Source: CAD feature listing. Evaluate the final solid. Frame: model axes, mm. Coordinates: 2 decimals unless noted, no trailing zeros. Order: outer loops, then holes, each group sorted by start corner. A loop starts at its lowest first (then second) coordinate and runs counter-clockwise, first axis right, second up.
Item 1: Section A-A on x = 0. Return the cut outline in (y, z), then the cut area to 3 significant figures.
Item 2: Section D-D on y = 101. Return the cut outline in (x, z).
Item 3: Section B-B on z = 3.5. State how many separate pieces and enclosed holes the cut face has, then the cut area to 3 significant figures.
Item 4: Section C-C on y = 0. Return the cut outline in (x, z).
Item 5: Mould query, pull axis Y, two halves, no side actions, for faces 1 (the cylindrical face through (6.154, -1.938, 3.131)), 2 (the cylindrical face through (-49.938, 320.133, 3.131)), 3 (the flat face through (-44, 161, 6.35)), 4 (the flat face through (-92.426, 381.018, 3.131)). Classes: released by +Y, released by -Y, zero draft, split by the parting line, or undercut.
Item 6: Ray query, line 1 (Y direction, x = -30, z = 4.75); line 2 (X direction, y = 71.5, z = 0.75); line 3 (X direction, y = 330.5, z = 2). Return the intervals inside material, ascending.
Autodesk Inventor part; units mm, degrees
ref_plane "Work Plane1" through (-0.0003, 0.0023, 0) normal (0, 0, 1) x (1, 0, 0)
ref_plane "YZ Plane" through (0, 0, 0) normal (1, 0, 0) x (0, 1, 0)
ref_plane "XZ Plane" through (0, 0, 0) normal (0, 1, 0) x (-1, 0, 0)
ref_plane "Work Plane1" through (-0.0003, 0.0023, 0) normal (0, 0, 1) x (1, 0, 0)
sketch "Sketch1" plane through (-0.0003, 0.0023, 0) normal (0, 0, 1) x (1, 0, 0)
  circle A0 centre (0.0003, -0.0023) radius 6.3373 construction
  circle A1 centre (-49.0975, 326.5271) radius 6.3373 construction
  circle A2 centre (0.0003, -0.0023) radius 6.4516
  circle A3 centre (-49.0975, 326.5271) radius 6.4516
  circle A4 centre (-49.0975, 326.5271) radius 60.325 construction
  circle A5 centre (0.0003, -0.0023) radius 60.325 construction
  circle A6 centre (0.0003, -0.0023) radius 31.75 construction
  line L0 (40.3672, -54.9357) -> (-26.6702, 390.9025)
  circle A7 centre (-49.0975, 326.5271) radius 31.75 construction
  line L1 (-58.7973, -69.8464) -> (40.3672, -54.9357)
  line L2 (-125.8347, 375.9918) -> (-26.6702, 390.9025)
  circle A8 centre (-54.0299, 68.9302) radius 6.3373 construction
  circle A9 centre (-36.6118, 251.3479) radius 6.3373 construction
  circle A10 centre (-54.0299, 68.9302) radius 6.4516
  line L3 (-82.6344, 131.3852) -> (-87.6899, 165.0073) construction
  line L4 (-58.7973, -69.8464) -> (-125.8347, 375.9918)
  point P0 (0.0003, -0.0023)
  dimension "d0" = 12.9032
  dimension "d3" = 12.9032
  dimension "d11" = 120.65
  dimension "d13" = 120.65
  dimension "d14" = 63.5
  dimension "d16" = 63.5
  dimension "d19" = 12.9032
extrude "Extrusion1" add sketch "Sketch1" along normal blind 6.35
sketch "Sketch2" plane through (-0.0003, 0.0023, 0) normal (0, 0, -1) x (-1, 0, 0)
  circle A0 centre (111.3879, 365.3242) radius 1.778 construction
  circle A1 centre (77.9428, 262.471) radius 1.778 construction
  circle A2 centre (31.0502, 180.1901) radius 1.778 construction
  circle A3 centre (64.857, 175.1068) radius 1.778 construction
  circle A4 centre (25.7636, 145.0307) radius 1.778 construction
  circle A5 centre (59.5704, 139.9475) radius 1.778 construction
  circle A6 centre (48.1268, -55.3992) radius 1.778 construction
  circle A7 centre (111.3879, 365.3242) radius 1.778
  circle A8 centre (77.9428, 262.471) radius 1.778
  circle A9 centre (64.857, 175.1068) radius 1.778
  circle A10 centre (59.5704, 139.9475) radius 1.778
  circle A11 centre (31.0502, 180.1901) radius 1.778
  circle A12 centre (25.7636, 145.0307) radius 1.778
  circle A13 centre (48.1268, -55.3992) radius 1.778
  point P0 (-0.0003, -0.0023)
extrude "Extrusion2" cut sketch "Sketch2" against normal through all
sketch "Sketch3" plane through (-0.0003, 0.0023, 0) normal (0, 0, -1) x (-1, 0, 0)
  circle A0 centre (-7.8664, -5.812) radius 2.8702 construction
  circle A1 centre (58.7683, 60.3758) radius 2.8702 construction
  circle A2 centre (41.3502, 242.7936) radius 2.8702
  circle A3 centre (41.2314, 320.7173) radius 2.8702 construction
  circle A4 centre (39.1236, 318.7692) radius 2.9567
  circle A5 centre (42.9235, 240.393) radius 2.8702
  circle A6 centre (60.507, 58.0922) radius 2.8702
  circle A7 centre (-10.0879, -7.6295) radius 2.8702
  point P0 (-0.0003, -0.0023)
extrude "Extrusion3" cut sketch "Sketch3" against normal through all contours A2 A5 | A2 A5 | A4 | A6 | A7 picked at (41.9477, 242.03) picked at (43.9052, 238.7756)
sketch "Sketch4" plane through (-0.0003, 0.0023, 0) normal (0, 0, -1) x (-1, 0, 0)
  arc A0 (58.0673, 386.1815) -> (21.1234, 354.0125) centre (58.7307, 348.1214) ccw construction
  arc A1 (58.0673, 386.1815) -> (21.1234, 354.0125) centre (58.7307, 348.1214) ccw
  line L0 (26.6702, 390.9025) -> (125.8347, 375.9918)
  line L1 (58.0673, 386.1815) -> (26.6702, 390.9025)
  line L2 (26.6702, 390.9025) -> (21.1234, 354.0125)
  point P0 (-0.0003, -0.0023)
extrude "Extrusion4" cut sketch "Sketch4" against normal through all
sketch "Sketch5" plane through (-0.0003, 0.0023, 0) normal (0, 0, -1) x (-1, 0, 0)
  circle A0 centre (-9.1502, 60.0002) radius 2.25 construction
  circle A1 centre (-9.1502, 60.0002) radius 1.8542
  point P0 (-0.0003, -0.0023)
  dimension "d30" = 3.7084
extrude "Extrusion5" cut sketch "Sketch5" against normal through all
sketch "Sketch6" plane through (-0.0003, 0.0023, 0) normal (0, 0, -1) x (-1, 0, 0)
  line L0 (-6.9196, 56.5789) -> (-27.6054, 48.4519) construction
  line L1 (-23.0039, 33.2159) -> (-17.622, 69.0087) construction
  line L2 (-40.3672, -54.9357) -> (21.1234, 354.0125) construction
  circle A0 centre (-19.2051, 50.473) radius 1.1906
  point P0 (-0.0003, -0.0023)
  dimension "d33" = 2.3813
extrude "Extrusion6" cut sketch "Sketch6" against normal through all
sketch "Sketch7" plane through (-0.0003, 0.0023, 0) normal (0, 0, -1) x (-1, 0, 0)
  circle A0 centre (32.9949, 251.8918) radius 6.3373 construction
  circle A1 centre (32.9949, 251.8918) radius 6.4516
  point P0 (-0.0003, -0.0023)
  dimension "d36" = 12.9032
extrude "Extrusion7" cut sketch "Sketch7" against normal through all
sketch "Sketch8" plane through (-0.0003, 0.0023, 0) normal (0, 0, -1) x (-1, 0, 0)
  circle A0 centre (91.5803, 211.0567) radius 3.81 construction
  circle A1 centre (79.685, 131.946) radius 3.81 construction
  circle A2 centre (48.0407, 136.7041) radius 3.81 construction
  circle A3 centre (59.936, 215.8148) radius 3.81 construction
  circle A4 centre (91.5803, 211.0567) radius 1.778
  circle A5 centre (79.685, 131.946) radius 1.778
  circle A6 centre (59.936, 215.8148) radius 1.778
  circle A7 centre (48.0407, 136.7041) radius 1.778
  point P0 (-0.0003, -0.0023)
  dimension "d39" = 3.556
  dimension "d40" = 3.556
  dimension "d41" = 3.556
  dimension "d42" = 3.556
extrude "Extrusion8" cut sketch "Sketch8" against normal through all
equation "\"d0\" = d3"
equation "\"d19\" = d3"
properties part number "inside wall"
Answer list:
1. outline: (-61, 0) - (-6.45, 0) - (-6.45, 6.35) - (-61, 6.35) - close; (6.45, 0) - (213.53, 0) - (213.53, 6.35) - (6.45, 6.35) - close
1. area: 1,660 mm2
2. outline: (-84.49, 0) - (16.92, 0) - (16.92, 6.35) - (-84.49, 6.35) - close
3. separate pieces: 1
3. enclosed holes: 21
3. area: 44,200 mm2
4. outline: (-69.3, 0) - (-6.45, 0) - (-6.45, 6.35) - (-69.3, 6.35) - close; (6.45, 0) - (32.11, 0) - (32.11, 6.35) - (6.45, 6.35) - close
5. face 1: undercut
5. face 2: undercut
5. face 3: zero draft
5. face 4: released by +Y
6. line 1: y = -65.51 to 178.76, 181.63 to 246.18, 257.61 to 373.09
6. line 2: x = -80.05 to -59.95, -48.11 to 21.36
6. line 3: x = -118.99 to -54.18, -44.01 to -17.59
